The listing builds one solid part. Answer for the finished solid, in the listing's coordinates (mm). A direction names the side the tool comes from. Give positions to 0.01 mm unless a question says otherwise; leave off trailing zeros. Write each loop counter-clockwise with the first axis right and the second up, starting at its lowest first coordinate (ties: lowest second). Pieces come first, ordered by that corner, then holes. Notation, with made-up numbers: (37.5, 47) - (68.5, 47) arc R22 cw to (68.5, 63) - close; hole circle Ø4 at (17.5, 6). An arc over 180 degrees is marked (long way). Answer in a Markdown table with one row per item. Add a question column.
from build123d import *

# Parameters (mm, degrees)
SKETCH_1_W          = 15.9
SKETCH_1_H          = 5.4
EXTRUDE_1_DEPTH     = 5.4
SKETCH_2_W          = 15.9
SKETCH_2_H          = 19.4
EXTRUDE_2_DEPTH     = 2
SKETCH_3_R          = 2.05
CUT_EXTRUDE_2_DEPTH = 14.654761074
CHAMFER_1_SIZE      = 1
FILLET_1_R          = 1


with BuildPart() as part:
    # 草图1 → 凸台-拉伸1 (new body)
    with BuildSketch(Plane(origin=(0, 0, 0), x_dir=(1, 0, 0), z_dir=(0, 1, 0))):
        Rectangle(SKETCH_1_W, SKETCH_1_H)
    extrude(amount=EXTRUDE_1_DEPTH)

    # 草图2 → 凸台-拉伸2 (add)
    with BuildSketch(Plane(origin=(0, 5.4, 0), x_dir=(1, 0, 0), z_dir=(0, 1, 0))):
        Rectangle(SKETCH_2_W, SKETCH_2_H)
    extrude(amount=EXTRUDE_2_DEPTH)

    # 草图3 → 切除-拉伸2 (cut, through all)
    with BuildSketch(Plane(origin=(0, 5.4, 0), x_dir=(-1, 0, 0), z_dir=(0, -1, 0))):
        with Locations(Location((0, 6.2, 0), (0, 0, 90))):
            Circle(SKETCH_3_R)
    cut_extrude_2 = extrude(amount=-CUT_EXTRUDE_2_DEPTH, mode=Mode.SUBTRACT)

    # 镜向2: 切除-拉伸2 across plane
    add(cut_extrude_2.mirror(Plane.XY), mode=Mode.SUBTRACT)

    # 倒角1
    chamfer_1_edges = [part.edges().sort_by_distance(p)[0] for p in [
        (0, 7.4, -4.15),
        (0, 7.4, 4.15),
    ]]
    chamfer(chamfer_1_edges, length=CHAMFER_1_SIZE)

    # 圆角1
    fillet_1_edges = [part.edges().sort_by_distance(p)[0] for p in [
        (0, 0, 2.7),
        (0, 0, -2.7),
    ]]
    fillet(fillet_1_edges, radius=FILLET_1_R)


solid = part.part
1. Section B-B (z = -6.2) is taken. Give the vertices of the cut face in (x, y).
2. A tool of negligible diameter and unlimited length cuts with its end or side. For faces 5 (the face through (0, 7.4, 0)), 6 (the face through (-2, 5.4, 5)), 7 (the face through (0, 3, -2.7)), from which of +Z, -Z, +X, -X, +Y, -Y can it reach the whole face along a straight path? Write none if from no direction.
3. Section A-A (x = 0) is taken. Give the vertices of the cut face in (y, z).
4. Section C-C (y = 6.75) is taken. Give the vertices of the cut face in (x, z), and give its area (3 significant figures).
5. The mould has two halves that part along Z. Classify faces 1 (the face through (0.616, 5.893, 8.155)), 2 (the face through (0, 5.4, -9)), 3 (the face through (0.616, 5.893, -8.155)), 4 (the face through (0, 3, 2.7)): +Z half, -Z half, draft (parallel to the pull), parting line (faces both ways), or undercut.
6. Section D-D (y = 1.75) is taken. Give the vertices of the cut face in (x, z), and give its area (3 significant figures).
7. Given pin 1 Ø7.5 at (x, z) = (-4, -5) entering from -Y; pin 2 Ø2 at (x, z) = (-0.5, 7.5) entering from -Y; pin 3 Ø2 at (x, y) = (4, 2.5) entering from -Z; pin 4 Ø1.5 at (x, y) = (5, 4.5) entering from +Z, each flat-ended and moving along its own axis, determine where each tip first touches the part or whether it passes through.
8. Straight lines are drawn through the part: L1, parallel to X at y = 6.05, z = 6.2; L2, parallel to Y at x = 5.75, z = -7.25; L3, parallel to Z at x = -1.75, y = 4.25. For each, find the intervals that lie inside material, in ascending order. Write a range as [from, to].
Geometry check:
| question | item | result |
|---|---|---|
| 1 | outline | (-7.95, 5.4) - (-2.05, 5.4) - (-2.05, 6.4) - (-3.05, 7.4) - (-7.95, 7.4) - close; (2.05, 5.4) - (7.95, 5.4) - (7.95, 7.4) - (3.05, 7.4) - (2.05, 6.4) - close |
| 2 | face 5 | +Z, -Z, +X, -X, +Y |
| 2 | face 6 | +Z, +X, -X, -Y |
| 2 | face 7 | -Z, +X, -X, -Y |
| 3 | outline | (0, -1.7) arc R1 ccw to (1, -2.7) - (5.4, -2.7) - (5.4, -4.15) - (6.4, -4.15) - (7.4, -3.15) - (7.4, 3.15) - (6.4, 4.15) - (5.4, 4.15) - (5.4, 2.7) - (1, 2.7) arc R1 ccw to (0, 1.7) - close; (5.4, -9.7) - (7.4, -9.7) - (7.4, -9.25) - (6.4, -8.25) - (5.4, -8.25) - close; (5.4, 8.25) - (6.4, 8.25) - (7.4, 9.25) - (7.4, 9.7) - (5.4, 9.7) - close |
| 4 | outline | (-7.95, -9.7) - (7.95, -9.7) - (7.95, 9.7) - (-7.95, 9.7) - close; hole circle Ø4.8 at (0, -6.2); hole circle Ø4.8 at (0, 6.2) |
| 4 | area | 272 mm² |
| 5 | face 1 | undercut |
| 5 | face 2 | draft |
| 5 | face 3 | undercut |
| 5 | face 4 | +Z half |
| 6 | outline | (-7.95, -2.7) - (7.95, -2.7) - (7.95, 2.7) - (-7.95, 2.7) - close |
| 6 | area | 85.9 mm² |
| 7 | pin 1 | y = 0 |
| 7 | pin 2 | y = 5.4 |
| 7 | pin 3 | z = -2.7 |
| 7 | pin 4 | z = 2.7 |
| 8 | L1 | [-7.95, -2.05], [2.05, 7.95] |
| 8 | L2 | [5.4, 7.4] |
| 8 | L3 | [-2.7, 2.7] |
